Job drawing, mm, ordinate dimensions from the low corner. One solid piece. A direction names the side the tool comes from. Coordinates: 2 decimals unless noted, no trailing zeros. Write each loop counter-clockwise with the first axis right and the second up, starting at its lowest first coordinate (ties: lowest second). Pieces come first, ordered by that corner, then holes. Notation, with made-up numbers: (22, 87.25) - (42, 87.25) arc R20 ccw to (42, 118.25) - close; hole circle Ø3 at (56, -37.75). An arc over 180 degrees is marked (long way). Use a Markdown table: item, result.
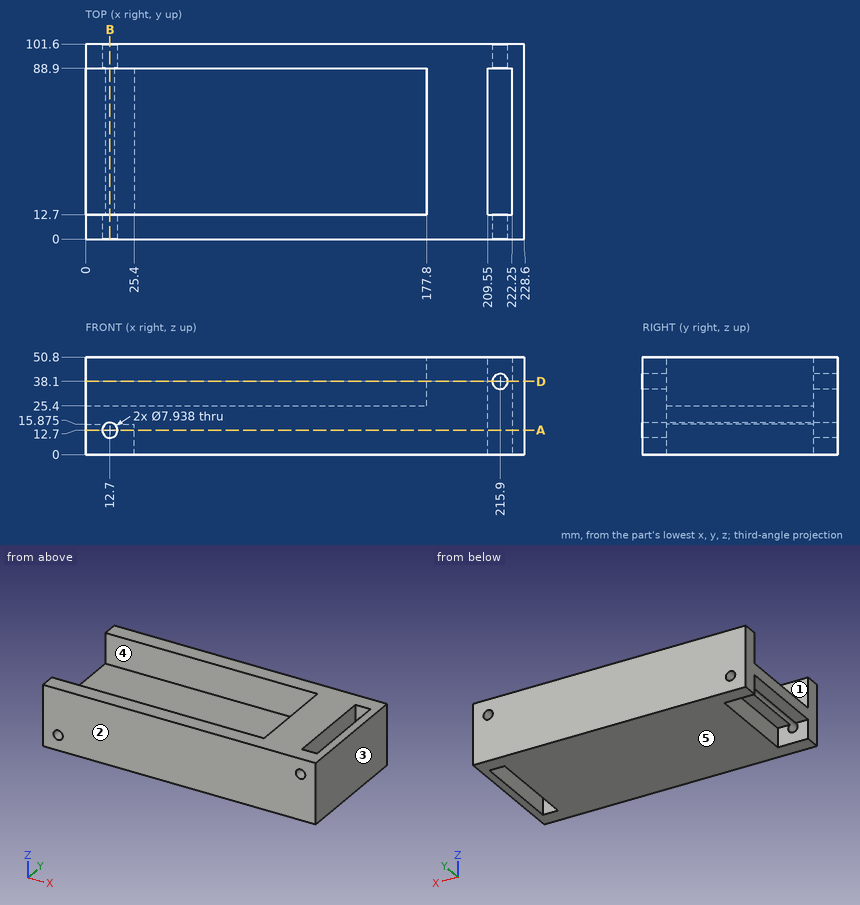
Item 1: Band-saw the part on B-B, the plane x = 12.7. Give the cut face in (y, z).
From the geometry:
| item | result |
|---|---|
| outline | (0, 0) - (12.7, 0) - (12.7, 8.73) - (0, 8.73) - close; (0, 16.67) - (101.6, 16.67) - (101.6, 50.8) - (88.9, 50.8) - (88.9, 25.4) - (12.7, 25.4) - (12.7, 50.8) - (0, 50.8) - close; (88.9, 0) - (101.6, 0) - (101.6, 8.73) - (88.9, 8.73) - close |
Item 2: Two-plate mould, pull along Y, no slides. Class the marked faces 1, 2 and 3: pulls with the +Y half, pulls with the -Y half, needs draft (parallel to the pull), parting line crosses it, or undercut.
From the geometry:
| item | result |
|---|---|
| face 1 | undercut |
| face 2 | pulls with the -Y half |
| face 3 | needs draft |
Item 3: Drill centre lines: probe 1 along X at (y, z) = (61.5, 24); probe 2 along Y at (x, z) = (73.5, 32.5); probe 3 along Z at (x, y) = (215.9, 9.5). Where is each one in solid material? Low to high.
From the geometry:
| item | result |
|---|---|
| probe 1 | 0 to 209.55, 222.25 to 228.6 |
| probe 2 | 0 to 12.7, 88.9 to 101.6 |
| probe 3 | 0 to 34.13, 42.07 to 50.8 |
Item 4: Which spindle directions (+Z, -Z, +X, -X, +Y, -Y) get a long thin tool onto all of the face, cutting with end or side? Do the marked faces 4 and 5. Say none if no direction does.
From the geometry:
| item | result |
|---|---|
| face 4 | +Z, -X |
| face 5 | -Z, +X, -X, +Y, -Y |
Item 5: Drop flat-ended pins along their axis: P1, Ø5, axis at y = 64.5, z = 7, coming from the -X side; P2, Ø12, axis at x = 198, z = 19, coming from the -Y side; P3, Ø11.5, axis at x = 18.5, y = 56.5, coming from the -Z side (1 decimal); P4, Ø6.5, axis at x = 215.9, z = 38.1, coming from the +Y side (3 decimals). Give the stop position or say it passes through.
From the geometry:
| item | result |
|---|---|
| P1 | x = 25.4 |
| P2 | y = 0 |
| P3 | z = 15.9 |
| P4 | through |
Item 6: Band-saw the part on D-D, the plane z = 38.1. Give the cut face in (x, y).
From the geometry:
| item | result |
|---|---|
| outline | (0, 0) - (211.93, 0) - (211.93, 12.7) - (209.55, 12.7) - (209.55, 88.9) - (211.93, 88.9) - (211.93, 101.6) - (0, 101.6) - (0, 88.9) - (177.8, 88.9) - (177.8, 12.7) - (0, 12.7) - close; (219.87, 0) - (228.6, 0) - (228.6, 101.6) - (219.87, 101.6) - (219.87, 88.9) - (222.25, 88.9) - (222.25, 12.7) - (219.87, 12.7) - close |
Item 7: Band-saw the part on A-A, the plane z = 12.7. Give the cut face in (x, y).
From the geometry:
| item | result |
|---|---|
| outline | (0, 0) - (8.73, 0) - (8.73, 12.7) - (0, 12.7) - close; (0, 88.9) - (8.73, 88.9) - (8.73, 101.6) - (0, 101.6) - close; (16.67, 0) - (228.6, 0) - (228.6, 101.6) - (16.67, 101.6) - (16.67, 88.9) - (25.4, 88.9) - (25.4, 12.7) - (16.67, 12.7) - close; hole (209.55, 12.7) - (222.25, 12.7) - (222.25, 88.9) - (209.55, 88.9) - close |
